Source: CAD feature listing. Evaluate the final solid. Frame: model axes, mm. A direction names the side the tool comes from. Give positions to 0.01 mm unless a question says otherwise; leave off trailing zeros. Loops run counter-clockwise (first coordinate to the right, second up) from the corner with the lowest first, then second, coordinate; pieces in that order, holes last. Notation, with made-up numbers: M 36,78.25 L 59,78.25 A20 ccw 59,88.25 Z; hole C 1,75.5 d11. An arc over 180 degrees is marked long. Answer in a Markdown table with one row per item.
```python
from build123d import *

# Parameters (mm, degrees)
F5_R      = 2.1
F6_DEPTH  = 30
F8_R      = 2.1
F9_DEPTH  = 30
F11_R     = 2.1
F12_DEPTH = 30
F13_R     = 1.25
F14_DEPTH = 8
F15_R     = 40


with BuildPart() as f1:
    # F0 (on Front) → F1 (revolve)
    with BuildSketch(Plane.XZ):
        Polygon((0, -2), (0, 0), (-18, 0), (-28.5, -28.8485129043), (-28.5, -40), (-22.5025773881, -40), (-15, -12), (-8, -12), (-8, -2), align=None)
    revolve(axis=Axis((0, 0, -1), (0, 0, -1)))

    # F5 (on face) → F6 (cut)
    with BuildSketch(Plane(origin=(0, -4.0048094716, -14.9461524227), x_dir=(1, 0, 0), z_dir=(0, 0.2588190451, 0.9659258263))):
        with Locations((0, -12.8830588531)):
            Circle(F5_R)
    extrude(amount=-F6_DEPTH, mode=Mode.SUBTRACT)

    # F8 (on face) → F9 (cut)
    with BuildSketch(Plane(origin=(-3.4682667397, 2.0024047358, -14.9461524227), x_dir=(0.9745560663, 0.0297636554, -0.2221589485), z_dir=(0.224143868, -0.1294095226, 0.9659258263))):
        with Locations((-11.0582542606, 6.6097063567)):
            Circle(F8_R)
    extrude(amount=-F9_DEPTH, mode=Mode.SUBTRACT)

    # F11 (on face) → F12 (cut)
    with BuildSketch(Plane(origin=(3.4682667397, 2.0024047358, -14.9461524227), x_dir=(0.9745560663, -0.0297636554, 0.2221589485), z_dir=(-0.224143868, -0.1294095226, 0.9659258263))):
        with Locations((11.0582542586, 6.6097063599)):
            Circle(F11_R)
    extrude(amount=-F12_DEPTH, mode=Mode.SUBTRACT)

    # F13 (on face) → F14 (cut)
    with BuildSketch(Plane(origin=(0, 0, -40), x_dir=(1, 0, 0), z_dir=(0, 0, -1))):
        with Locations((-22.5166604984, 13)):
            Circle(F13_R)
        with Locations((22.5166604984, 13)):
            Circle(F13_R)
        with Locations((0, -26)):
            Circle(F13_R)
    extrude(amount=-F14_DEPTH, mode=Mode.SUBTRACT)

    # F15
    f15_edges = [f1.edges().sort_by_distance(p)[0] for p in [
        (28.5, 0, -28.848513),
    ]]
    fillet(f15_edges, radius=F15_R)


solid = f1.part
```
1) Pin query (flat end, axial travel): pin 1 Ø13 at (x, y) = (0, 0) entering from -Z; pin 2 Ø9 at (x, y) = (-3, -5) entering from -Z; pin 3 Ø10 at (x, z) = (17.5, -21.5) entering from +Y. Return the tip coordinate at first contact, or that it passes through.
Reply:
| item | result |
|---|---|
| pin 1 | stops at z = -2 |
| pin 2 | stops at z = -12 |
| pin 3 | stops at y = 23.21 |
2) Set-up query: faces 4 (the flat face through (22, -13, -32)), 5 (the conical face through (-18.51, 5.83, -3.86)), 6 (the flat face through (14.24, 8.25, -11.61)). Return all of +Z, -Z, +X, -X, +Y, -Y with unobstructed straight access to the full face (end or side cutting, diameter ignored); none if empty.
Reply:
| item | result |
|---|---|
| face 4 | -Z |
| face 5 | +Z |
| face 6 | none |
3) Material intervals for L1, parallel to Y at x = 0, z = -33.75; L2, parallel to X at y = -10, z = -35.5; L3, parallel to X at y = -13, z = -35, sorted ascending.
Reply:
| item | result |
|---|---|
| L1 | y = -28.44 to -24.55, 20.83 to 24.75, 27.25 to 28.44 |
| L2 | x = -26.69 to -18.8, 18.8 to 26.69 |
| L3 | x = -25.35 to -23.77, -21.27 to -16.7, 16.7 to 21.27, 23.77 to 25.35 |
4) Section A-A, the plane z = -8.5. Return loops of the section in (x, y), then the cut area to 3 significant figures.
Reply:
| item | result |
|---|---|
| outline | C 0,0 d42.19; hole C 0,0 d16 |
| area | 1,200 mm² |
5) Pull-direction query (Y, two-part tool) for faces 1 (the flat face through (13, -19, -40)), 2 (the cylindrical face through (-26.327, -10.916, -37.979)), 3 (the flat face through (0, 26, -32)); classes: released by +Y, released by -Y, zero draft, split by the parting line, or undercut.
Reply:
| item | result |
|---|---|
| face 1 | zero draft |
| face 2 | split by the parting line |
| face 3 | undercut |
